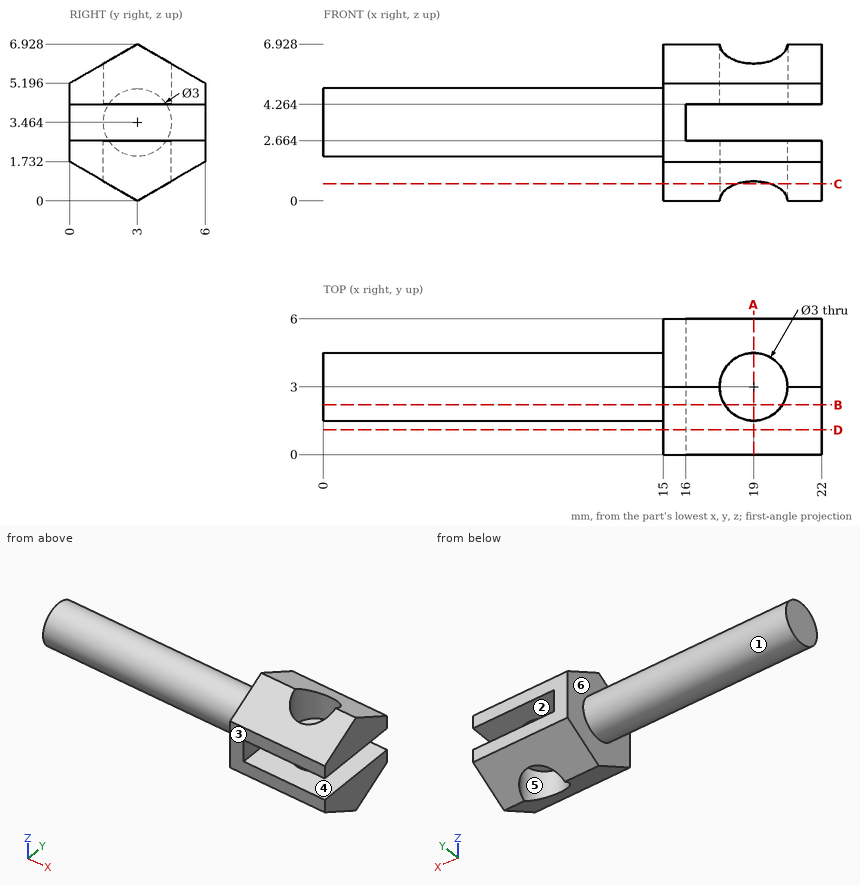
Geometry check sheet. Reference: drawing and pictorial views, mm from the part's lowest x, y, z. A direction names the side the tool comes from. Give positions to 0.01 mm unless a question says otherwise; leave off trailing zeros. Order: outer loops, then holes, each group sorted by start corner. A loop starts at its lowest first (then second) coordinate and runs counter-clockwise, first axis right, second up. Notation, with made-up numbers: M 17.5,-14.5 L 43.5,-14.5 A27 ccw 43.5,3.5 Z; hole C 10,64 d11. An arc over 180 degrees is marked long. Answer in a Markdown table with one row per item. Add a question column.
Q1. Sectioned sample at B-B, the plane y = 2.2. Record the boundary of the cut face in (x, z) (1 decimal).
Q2. Sectioned sample at D-D, the plane y = 1.1. Record the boundary of the cut face in (x, z).
Q3. Release check for a two-part mould opening along Z. For the marked faces 1, 2 and 3 record: released by +Z, released by -Z, zero draft, split by the parting line, or undercut.
Q4. Access from +Z, -Z, +X, -X, +Y, -Y to the whole of each face (thin tool, end or side, straight path). Record for the marked faces 4, 5 and 6.
Q5. Thickness scan on L1, parallel to X at y = 3, z = 0.7; L2, parallel to Y at x = 19, z = 5.05; L3, parallel to X at y = 2.85, z = 4. Record the ranges inside material, lowest first.
Q6. Sectioned sample at A-A, the plane x = 19. Record the boundary of the cut face in (y, z).
Q7. Sectioned sample at C-C, the plane z = 0.75. Record the boundary of the cut face in (x, y).
Q8. Gauge pin test, flat ends, axial feed: pin 1 Ø2 at (x, y) = (18, 5) entering from -Z; pin 2 Ø2.5 at (x, y) = (19, 3) entering from -Z; pin 3 Ø4 at (x, z) = (8.5, 3.5) entering from +Y. Record the tip position at first contact, or that the pin passes through.
Verdict:
| question | item | result |
|---|---|---|
| 1 | outline | M 0,2.2 L 15,2.2 L 15,0.5 L 17.7,0.5 L 17.7,2.7 L 16,2.7 L 16,4.3 L 17.7,4.3 L 17.7,6.5 L 15,6.5 L 15,4.7 L 0,4.7 Z; M 20.3,0.5 L 22,0.5 L 22,2.7 L 20.3,2.7 Z; M 20.3,4.3 L 22,4.3 L 22,6.5 L 20.3,6.5 Z |
| 2 | outline | M 15,1.1 L 22,1.1 L 22,2.66 L 16,2.66 L 16,4.26 L 22,4.26 L 22,5.83 L 15,5.83 Z |
| 3 | face 1 | split by the parting line |
| 3 | face 2 | undercut |
| 3 | face 3 | zero draft |
| 4 | face 4 | +X, +Y, -Y |
| 4 | face 5 | +Z, -Z |
| 4 | face 6 | -X |
| 5 | L1 | 15 to 17.5, 20.5 to 22 |
| 5 | L2 | 0 to 1.5, 4.5 to 6 |
| 5 | L3 | 0 to 16 |
| 6 | outline | M 0,1.73 L 1.5,0.87 L 1.5,2.66 L 0,2.66 Z; M 0,4.26 L 1.5,4.26 L 1.5,6.06 L 0,5.2 Z; M 4.5,0.87 L 6,1.73 L 6,2.66 L 4.5,2.66 Z; M 4.5,4.26 L 6,4.26 L 6,5.2 L 4.5,6.06 Z |
| 7 | outline | M 15,1.7 L 18.25,1.7 A1.5 cw 18.25,4.3 L 15,4.3 Z; M 19.75,1.7 L 22,1.7 L 22,4.3 L 19.75,4.3 A1.5 cw Z |
| 8 | pin 1 | z = 0.58 |
| 8 | pin 2 | through |
| 8 | pin 3 | y = 4.5 |
